Work out the finished part from the listing and answer in its coordinate system (mm). Give positions to 0.01 mm unless a question says otherwise; leave off trailing zeros. Order: outer loops, then holes, each group sorted by start corner. A loop starts at its lowest first (then second) coordinate and runs counter-clockwise, first axis right, second up. Notation, with made-up numbers: M 15.5,59.5 L 36.5,59.5 A29 cw 36.5,91.5 Z; hole C 54,49 d4. An arc over 180 degrees is marked long. One line per item, written item: value.
Autodesk Inventor part; units mm, degrees
ref_plane "YZ Plane" through (0, 0, 0) normal (1, 0, 0) x (0, 1, 0)
ref_plane "XZ Plane" through (0, 0, 0) normal (0, 1, 0) x (-1, 0, 0)
ref_plane "XY Plane" through (0, 0, 0) normal (0, 0, 1) x (1, 0, 0)
sketch "Skizze1" plane through (0, 0, 0) normal (0, 1, 0) x (-1, 0, 0)
  line L0 (0, 0) -> (90.25, 0)
  line L1 (90.25, 0) -> (90.25, 57.5)
  line L2 (90.25, 57.5) -> (0, 57.5)
  line L3 (0, 57.5) -> (0, 0)
  dimension "d0" = 90.25
  dimension "d1" = 57.5
extrude "Extrusion1" add sketch "Skizze1" along normal blind 16.5
hole "Bohrung1" at (-16.5, 0, 28.75) direction (0, 1, 0) diameter 4 end through all
hole "Bohrung2" at (-73.75, 0, 28.75) direction (0, 1, 0) diameter 4 end through all
properties part number "Batteriehalter_6AA" material "PBT-Kunststoff"
(1) Given P1, Ø2.5, axis at x = -73.75, z = 28.75, coming from the -Y side, flat-ended and moving along its own axis, determine where the tip first touches the part or whether it passes through.
Findings:
P1: passes through
(2) Section A-A, the plane x = -16.5 is taken. Give the vertices of the cut face in (y, z).
Findings:
outline: M 0,0 L 16.5,0 L 16.5,26.75 L 0,26.75 Z; M 0,30.75 L 16.5,30.75 L 16.5,57.5 L 0,57.5 Z
(3) Determine the mould class of faces 1 (the flat face through (0, 8, 29)), 2 (the cylindrical face through (-75.436, 8.366, 27.675)), 3 (the flat face through (-46, 8, 57.5)) for opening direction X: pulls with the +X half, pulls with the -X half, needs draft (parallel to the pull), parting line crosses it, or undercut.
Findings:
face 1: pulls with the +X half
face 2: undercut
face 3: needs draft
(4) Section B-B, the plane z = 28.75 is taken. Give the vertices of the cut face in (x, y).
Findings:
outline: M -90.25,0 L -75.75,0 L -75.75,16.5 L -90.25,16.5 Z; M -71.75,0 L -18.5,0 L -18.5,16.5 L -71.75,16.5 Z; M -14.5,0 L 0,0 L 0,16.5 L -14.5,16.5 Z
(5) Find the intervals of material crossed by probe 1 along X at (y, z) = (12.25, 28.75); probe 2 along Z at (x, y) = (-16.5, 10.25); probe 3 along X at (y, z) = (15.5, 30.5), in increasing order. Write a range as from..to.
Findings:
probe 1: x = -90.25..-75.75, -71.75..-18.5, -14.5..0
probe 2: z = 0..26.75, 30.75..57.5
probe 3: x = -90.25..-74.72, -72.78..-17.47, -15.53..0
